Verification items for the finished model (mm, model axes). Face numbers are marked on the shaded views. A direction names the side the tool comes from. Give positions to 0.01 mm unless a question says otherwise; leave off trailing zeros. Order: outer loops, then holes, each group sorted by start corner. A loop starts at its lowest first (then second) coordinate and runs counter-clockwise, first axis right, second up. Notation, with made-up numbers: (51.25, 88) - (73.25, 88) arc R15 cw to (73.25, 107) - close; hole circle Ø7 at (-31, 67.25). An arc over 180 degrees is marked (long way). Answer as a JSON object with one key per item and string values.
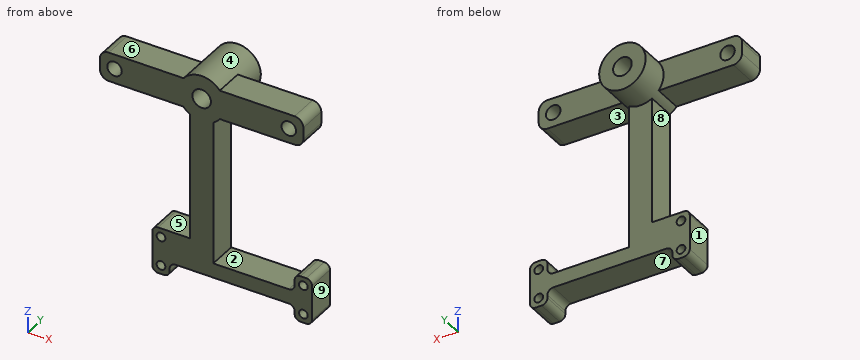
```python
from build123d import *

# Parameters (mm, degrees)
SKETCH_2_W           = 8
SKETCH_2_H           = 17
EXTRUDE_1_DEPTH      = 10
SKETCH_4_R           = 3.2
SKETCH_4_R_2         = 2.5
EXTRUDE_2_DEPTH      = 10
SKETCH_6_R           = 1.5
EXTRUDE_3_DEPTH      = 10
FILLET_6_R           = 2
FILLET_7_R           = 3
EXTRUDE_4_DEPTH      = 10
EXTRUDE_4_DEPTH_BACK = 10
SKETCH_7_R           = 8
SKETCH_7_R_2         = 3.2


with BuildPart() as part:
    # Sketch 2 → Extrude 1 (new body)
    with BuildSketch(Plane(origin=(0, 0, 0), x_dir=(1, 0, 0), z_dir=(0, 1, 0))):
        with Locations((0, -14.5)):
            Rectangle(SKETCH_2_W, SKETCH_2_H)
    extrude(amount=EXTRUDE_1_DEPTH)

    # Sketch 4 → Extrude 2 (add)
    with BuildSketch(Plane(origin=(0, 10, 0), x_dir=(1, 0, 0), z_dir=(0, 1, 0))):
        Polygon((-4, -23), (4, -23), (4, -61.531911565), (35, -61.531911565), (35, -71.531911565), (-35, -71.531911565), (-35, -61.531911565), (-4, -61.531911565), align=None)
        with Locations(Location((0, -66.5, 0), (0, 0, 270))):
            Circle(SKETCH_4_R, mode=Mode.SUBTRACT)
        with Locations(Location((30, -66.5, 0), (0, 0, 270))):
            Circle(SKETCH_4_R_2, mode=Mode.SUBTRACT)
        with Locations(Location((-30, -66.5, 0), (0, 0, 270))):
            Circle(SKETCH_4_R_2, mode=Mode.SUBTRACT)
    extrude(amount=-EXTRUDE_2_DEPTH)

    # Sketch 6 → Extrude 3 (add)
    with BuildSketch(Plane(origin=(0, 10, 0), x_dir=(1, 0, 0), z_dir=(0, 1, 0))):
        Polygon((-17, 0), (-17, -16), (-4, -16), (-4, -10), (32, -10), (32, -16), (38, -16), (38, 0), (32, 0), (32, -5), (-11, -5), (-11, 0), align=None)
        with Locations(Location((-14, -3, 0), (0, 0, 270))):
            Circle(SKETCH_6_R, mode=Mode.SUBTRACT)
        with Locations(Location((-14, -13, 0), (0, 0, 270))):
            Circle(SKETCH_6_R, mode=Mode.SUBTRACT)
        with Locations(Location((35, -3, 0), (0, 0, 270))):
            Circle(SKETCH_6_R, mode=Mode.SUBTRACT)
        with Locations(Location((35, -13, 0), (0, 0, 270))):
            Circle(SKETCH_6_R, mode=Mode.SUBTRACT)
    extrude(amount=-EXTRUDE_3_DEPTH)

    # Fillet 6
    fillet_6_edges = [part.edges().sort_by_distance(p)[0] for p in [
        (32, 5, 10),
        (-17, 5, 0),
        (-11, 5, 0),
        (-11, 5, 5),
        (32, 5, 5),
        (32, 5, 0),
        (38, 5, 0),
        (38, 5, 16),
        (32, 5, 16),
        (-17, 5, 16),
    ]]
    fillet(fillet_6_edges, radius=FILLET_6_R)

    # Fillet 7
    fillet_7_edges = [part.edges().sort_by_distance(p)[0] for p in [
        (35, 5, 61.531911565),
        (35, 5, 71.531911565),
        (-35, 5, 71.531911565),
        (-35, 5, 61.531911565),
    ]]
    fillet(fillet_7_edges, radius=FILLET_7_R)

    # Sketch 7 → Extrude 4 (add, two sides: drawn at the far end of the back side and taken through both)
    with BuildSketch(Plane(origin=(0, 10, 0), x_dir=(1, 0, 0), z_dir=(0, 1, 0)).offset(-EXTRUDE_4_DEPTH_BACK)):
        with Locations(Location((0, -66.5, 0), (0, 0, 270))):
            Circle(SKETCH_7_R)
        with Locations(Location((0, -66.5, 0), (0, 0, 270))):
            Circle(SKETCH_7_R_2, mode=Mode.SUBTRACT)
    extrude(amount=EXTRUDE_4_DEPTH + EXTRUDE_4_DEPTH_BACK)


solid = part.part
```
(1) Gauge pin test, flat ends, axial feed: pin 1 Ø5 at (x, z) = (23.5, 66.5) entering from +Y; pin 2 Ø12 at (x, y) = (29.5, 15.5) entering from +Z; pin 3 Ø5 at (y, z) = (3.5, 11) entering from -X. Record the tip position at first contact, or that the pin passes through.
Computed values:
{"pin 1": "stops at y = 10", "pin 2": "stops at z = 71.53", "pin 3": "stops at x = -17"}
(2) Release check for a two-part mould opening along X. For the marked faces 6, 7, 8 and 9 record: pulls with the +X half, pulls with the -X half, needs draft (parallel to the pull), parting line crosses it, or undercut.
Computed values:
{"face 6": "needs draft", "face 7": "undercut", "face 8": "pulls with the -X half", "face 9": "pulls with the +X half"}
(3) Access from +Z, -Z, +X, -X, +Y, -Y to the whole of each face (thin tool, end or side, straight path). Record for the marked faces 1, 2, 3, 4 and 5.
Computed values:
{"face 1": "-Z, -X, +Y, -Y", "face 2": "+Y, -Y", "face 3": "+X, +Y, -Y", "face 4": "+Y", "face 5": "-X, +Y, -Y"}
(4) Section check C-C (x = -14). Record the cut outline in (y, z).
Computed values:
{"outline": "(0, 0) - (10, 0) - (10, 1.5) - (0, 1.5) - close; (0, 4.5) - (10, 4.5) - (10, 11.5) - (0, 11.5) - close; (0, 14.5) - (10, 14.5) - (10, 16) - (0, 16) - close; (0, 61.53) - (10, 61.53) - (10, 71.53) - (0, 71.53) - close"}
(5) Section check D-D (z = 22). Record the cut outline in (x, y).
Computed values:
{"outline": "(-4, 0) - (4, 0) - (4, 10) - (-4, 10) - close"}
(6) Material ranges on line 1 along X through (y, z) = (13.75, 66.5); line 2 along Y through (x, z) = (-7.5, 8); line 3 along Z through (x, y) = (7, 2), recorded low to high. Write a range as [from, to].
Computed values:
{"line 1": "x = [-8, -3.2], [3.2, 8]", "line 2": "y = [0, 10]", "line 3": "z = [5, 10], [61.53, 71.53]"}
(7) Section check A-A (x = 22). Record the cut outline in (y, z).
Computed values:
{"outline": "(0, 5) - (10, 5) - (10, 10) - (0, 10) - close; (0, 61.53) - (10, 61.53) - (10, 71.53) - (0, 71.53) - close"}
(8) Section check B-B (z = 13). Record the cut outline in (x, y).
Computed values:
{"outline": "(-17, 0) - (-15.5, 0) - (-15.5, 10) - (-17, 10) - close; (-12.5, 0) - (4, 0) - (4, 10) - (-12.5, 10) - close; (32, 0) - (33.5, 0) - (33.5, 10) - (32, 10) - close; (36.5, 0) - (38, 0) - (38, 10) - (36.5, 10) - close"}
